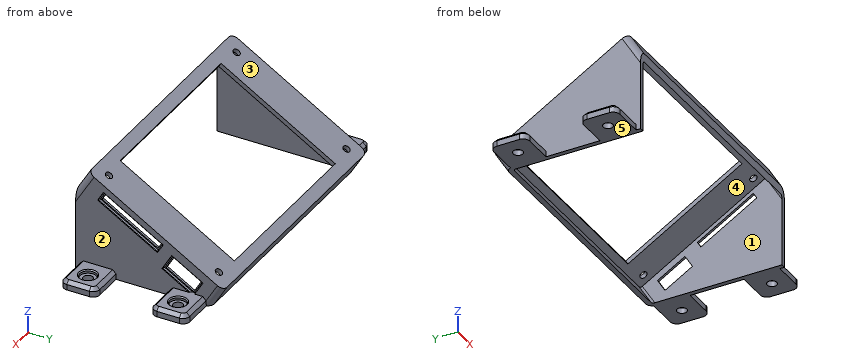
from build123d import *

# Parameters (mm, degrees)
BOSS_EXTRUDE1_DEPTH      = 115
SKETCH2_W                = 115
SKETCH2_H                = 70
BOSS_EXTRUDE2_DEPTH      = 11
FILLET1_R                = 3
SHELL1_T                 = -2
SKETCH3_R                = 1.6
CUT_EXTRUDE1_DEPTH       = 2
SKETCH4_W                = 80.6
SKETCH4_H                = 59.2
CUT_EXTRUDE2_DEPTH       = 2
CUT_EXTRUDE3_DEPTH       = 2
CUT_EXTRUDE4_DEPTH       = 1
CHAMFER3_SIZE            = 0.5
BOSS_EXTRUDE3_START      = -2
SKETCH7_W                = 4
SKETCH7_H                = 16
BOSS_EXTRUDE3_DEPTH      = 18
SKETCH8_R                = 2.125
CUT_EXTRUDE5_DEPTH       = 4
SKETCH9_R                = 3.65
CUT_EXTRUDE6_DEPTH       = 1.5
CHAMFER4_SIZE            = 0.5
FILLET2_R                = 3
CHAMFER4_OF_MIRROR1_SIZE = 0.5
FILLET2_OF_MIRROR1_R     = 3
CHAMFER5_SIZE            = 1.5


with BuildPart() as part:
    # Sketch1 → Boss-Extrude1 (new body)
    with BuildSketch(Plane(origin=(0, 0, 0), x_dir=(0, 0, -1), z_dir=(1, 0, 0))):
        Polygon((0, 0), (0, 60), (-36.055512755, 0), align=None)
    extrude(amount=BOSS_EXTRUDE1_DEPTH)

    # Sketch2 → Boss-Extrude2 (add)
    with BuildSketch(Plane(origin=(0, 15.918367347, 26.489764473), x_dir=(1, 0, 0), z_dir=(0, 0.515078754, 0.857142857))):
        with Locations((57.5, 16.428571429)):
            Rectangle(SKETCH2_W, SKETCH2_H)
    extrude(amount=BOSS_EXTRUDE2_DEPTH)

    # Fillet1
    fillet1_edges = [part.edges().sort_by_distance(p)[0] for p in [
        (0, 62.832933145, 4.714285714),
        (0, 2.832933145, 40.769798469),
        (115, 2.832933145, 40.769798469),
        (115, 62.832933145, 4.714285714),
    ]]
    fillet(fillet1_edges, radius=FILLET1_R)

    # Shell1
    shell1_openings = [part.faces().sort_by_distance(p)[0] for p in [
        (57.5, 39.074957911, 0),
        (57.5, 0, 22.497645419),
    ]]
    offset(amount=SHELL1_T, openings=shell1_openings, kind=Kind.INTERSECTION)

    # Sketch3 → Cut-Extrude1 (cut)
    with BuildSketch(Plane(origin=(0, 21.584233637, 35.918335901), x_dir=(1, 0, 0), z_dir=(0, 0.515078754, 0.857142857))):
        with Locations((6.5, 44.928571429)):
            Circle(SKETCH3_R)
        with Locations((6.5, -12.071428571)):
            Circle(SKETCH3_R)
        with Locations((108.5, -12.071428571)):
            Circle(SKETCH3_R)
        with Locations((108.5, 44.928571429)):
            Circle(SKETCH3_R)
    extrude(amount=-CUT_EXTRUDE1_DEPTH, mode=Mode.SUBTRACT)

    # Sketch4 → Cut-Extrude2 (cut)
    with BuildSketch(Plane(origin=(0, 21.584233637, 35.918335901), x_dir=(1, 0, 0), z_dir=(0, 0.515078754, 0.857142857))):
        with Locations((57.5, 16.428571429)):
            Rectangle(SKETCH4_W, SKETCH4_H)
    extrude(amount=-CUT_EXTRUDE2_DEPTH, mode=Mode.SUBTRACT)

    # Sketch5 → Cut-Extrude3 (cut)
    with BuildSketch(Plane(origin=(115, 0, 0), x_dir=(0, 0, -1), z_dir=(1, 0, 0))):
        Polygon((-36.861471556, 12.734320964), (-34.290042984, 11.189084703), (-19.352759129, 36.04622756), (-21.9241877, 37.591463821), align=None)
        Polygon((-17.207652396, 43.110512174), (-9.872930944, 55.31622646), (-4.301502372, 51.968214561), (-11.636223824, 39.762500275), align=None)
    extrude(amount=-CUT_EXTRUDE3_DEPTH, mode=Mode.SUBTRACT)

    # Sketch6 → Cut-Extrude4 (cut)
    with BuildSketch(Plane(origin=(115, 0, 0), x_dir=(0, 0, -1), z_dir=(1, 0, 0))):
        Polygon((-38.233693167, 12.39225686), (-33.947978881, 9.816863092), (-17.980537518, 36.388291664), (-22.266251804, 38.963685432), align=None)
        Polygon((-11.294159721, 38.390278664), (-2.929280762, 52.310278664), (-10.214995047, 56.68844807), (-18.579874006, 42.76844807), align=None)
    extrude(amount=-CUT_EXTRUDE4_DEPTH, mode=Mode.SUBTRACT)

    # Chamfer3
    chamfer3_edges = [part.edges().sort_by_distance(p)[0] for p in [
        (114, 40.579363367, 14.937016864),
        (114, 49.72844807, 14.397434527),
        (114, 54.499363367, 6.572137904),
        (114, 45.350278664, 7.111720241),
        (114, 25.677971146, 30.249972485),
        (114, 37.675988548, 20.123394661),
        (114, 23.102577378, 25.964258199),
        (114, 11.104559976, 36.090836024),
    ]]
    chamfer(chamfer3_edges, length=CHAMFER3_SIZE)

    # Sketch7 → Boss-Extrude3 (add)
    with BuildSketch(Plane(origin=(115, 0, 0), x_dir=(0, 0, -1), z_dir=(1, 0, 0)).offset(BOSS_EXTRUDE3_START)):
        with Locations((-2, 50)):
            Rectangle(SKETCH7_W, SKETCH7_H)
        with Locations((-2, 10)):
            Rectangle(SKETCH7_W, SKETCH7_H)
    boss_extrude3 = extrude(amount=BOSS_EXTRUDE3_DEPTH)

    # Sketch8 → Cut-Extrude5 (cut)
    with BuildSketch(Plane.XY.offset(4)):
        with Locations((123, 50)):
            Circle(SKETCH8_R)
        with Locations((123, 10)):
            Circle(SKETCH8_R)
    cut_extrude5 = extrude(amount=-CUT_EXTRUDE5_DEPTH, mode=Mode.SUBTRACT)

    # Sketch9 → Cut-Extrude6 (cut)
    with BuildSketch(Plane.XY.offset(4)):
        with Locations((123, 50)):
            Circle(SKETCH9_R)
        with Locations((123, 10)):
            Circle(SKETCH9_R)
    cut_extrude6 = extrude(amount=-CUT_EXTRUDE6_DEPTH, mode=Mode.SUBTRACT)

    # Chamfer4
    chamfer4_edges = [part.edges().sort_by_distance(p)[0] for p in [
        (119.35, 50, 4),
        (119.35, 10, 4),
    ]]
    chamfer(chamfer4_edges, length=CHAMFER4_SIZE)

    # Fillet2
    fillet2_edges = [part.edges().sort_by_distance(p)[0] for p in [
        (131, 58, 2),
        (131, 42, 2),
        (131, 18, 2),
        (131, 2, 2),
    ]]
    fillet(fillet2_edges, radius=FILLET2_R)

    # Mirror1: Boss-Extrude3, Cut-Extrude5, Cut-Extrude6 across plane
    add(boss_extrude3.mirror(Plane(origin=(57.5, 0, 0), x_dir=(0, 0, 1), z_dir=(1, 0, 0))))
    add(cut_extrude5.mirror(Plane(origin=(57.5, 0, 0), x_dir=(0, 0, 1), z_dir=(1, 0, 0))), mode=Mode.SUBTRACT)
    add(cut_extrude6.mirror(Plane(origin=(57.5, 0, 0), x_dir=(0, 0, 1), z_dir=(1, 0, 0))), mode=Mode.SUBTRACT)

    # Chamfer4 of Mirror1
    chamfer4_of_mirror1_edges = [part.edges().sort_by_distance(p)[0] for p in [
        (-4.35, 50, 4),
        (-4.35, 10, 4),
    ]]
    chamfer(chamfer4_of_mirror1_edges, length=CHAMFER4_OF_MIRROR1_SIZE)

    # Fillet2 of Mirror1
    fillet2_of_mirror1_edges = [part.edges().sort_by_distance(p)[0] for p in [
        (-16, 58, 2),
        (-16, 42, 2),
        (-16, 18, 2),
        (-16, 2, 2),
    ]]
    fillet(fillet2_of_mirror1_edges, radius=FILLET2_OF_MIRROR1_R)

    # Chamfer5
    chamfer5_edges = [part.edges().sort_by_distance(p)[0] for p in [
        (121.5, 42, 4),
        (121.5, 58, 4),
        (121.5, 2, 4),
        (121.5, 18, 4),
        (131, 10, 4),
        (130.121320344, 2.878679656, 4),
        (130.121320344, 17.121320344, 4),
        (131, 50, 4),
        (130.121320344, 42.878679656, 4),
        (130.121320344, 57.121320344, 4),
        (-6.5, 58, 4),
        (-6.5, 42, 4),
        (-6.5, 18, 4),
        (-6.5, 2, 4),
        (-16, 10, 4),
        (-15.121320344, 2.878679656, 4),
        (-15.121320344, 17.121320344, 4),
        (-16, 50, 4),
        (-15.121320344, 42.878679656, 4),
        (-15.121320344, 57.121320344, 4),
    ]]
    chamfer(chamfer5_edges, length=CHAMFER5_SIZE)


solid = part.part
Geometry: final body of the model. Coordinates: model frame, mm. Face numbers are marked on the shaded views. A direction names the side the tool comes from. Give positions to 0.01 mm unless a question says otherwise; leave off trailing zeros. Loops run counter-clockwise (first coordinate to the right, second up) from the corner with the lowest first, then second, coordinate; pieces in that order, holes last. Notation, with made-up numbers: M 58,14 L 69,14 A35 ccw 69,53 Z; hole C -20,74.25 d4. An arc over 180 degrees is marked long. Put each result on its own line as item: value. Start each with the question number.
1) Cut plane A-A (x = -8). Give the number of separate pieces and of enclosed holes in the cut face, then the cut area to 4 significant figures.
2) Access query for the marked faces 4 and 5. Directions: +Z, -Z, +X, -X, +Y, -Y. A direction counts if a zero-diameter tool reaches every point of the face in a straight line with its end or side. Return the directions, or none.
3) Cut plane C-C (x = 94.5). Output: boundary loops of the cut face in (y, z), then the cut area to 3 significant figures.
4) Contact query for flat-ended pins moving along their axis: pin 1 (6 mm diameter, centred on x = 123, y = 9.5, fed in from +Z); pin 2 (4.5 mm diameter, centred on x = -8, y = 50, fed in from -Z); pin 3 (1.5 mm diameter, centred on x = 8.5, y = 47, fed in from -Z); pin 4 (2 mm diameter, centred on y = 56.5, z = 6.5, fed in from +X). Output: stop coordinate, or through.
5) Cut plane B-B (x = 116.5). Output: boundary loops of the cut face in (y, z), then the cut area to 4 significant figures.
6) Pull-direction query (X, two-part tool) for the marked faces 1, 2 and 3; classes: pulls with the +X half, pulls with the -X half, needs draft (parallel to the pull), parting line crosses it, or undercut.
7) Ray query, line 1 along Y through (x, z) = (123, 1.4) (3 decimals); line 2 along X through (y, z) = (37.5, 17.5); line 3 along X through (y, z) = (40, 23.5). Return the intervals inside material, ascending.
Verdict:
1. separate pieces: 4
1. enclosed holes: 0
1. area: 79.85 mm2
2. face 4: none
2. face 5: -Z, +X, -X, +Y, -Y
3. outline: M 0,32.17 L 6.35,42.74 L 9.26,40.99 L 10.29,42.7 L 5.67,45.48 L 0,36.06 Z; M 57.67,0 L 60,0 L 65.67,9.43 L 61.04,12.21 L 60.01,10.5 L 62.92,8.74 Z
3. area: 62.1 mm2
4. pin 1: z = 2.5
4. pin 2: z = 0
4. pin 3: z = 17.86
4. pin 4: x = 115
5. outline: M 2,0 L 18,0 L 18,2.5 L 16.5,4 L 3.5,4 L 2,2.5 Z; M 42,0 L 58,0 L 58,2.5 L 56.5,4 L 43.5,4 L 42,2.5 Z
5. area: 123.5 mm2
6. face 1: undercut
6. face 2: pulls with the +X half
6. face 3: needs draft
7. line 1: 2 to 7.875, 12.125 to 18, 42 to 47.875, 52.125 to 58
7. line 2: 0 to 2, 113 to 115
7. line 3: 0 to 17.2, 97.8 to 115
